Verification items for the finished model (mm, model axes). A direction names the side the tool comes from. Round coordinates to 2 decimals unless told otherwise and drop trailing zeros. Loops run counter-clockwise (first coordinate to the right, second up) from the corner with the lowest first, then second, coordinate; pieces in that order, holes last. Notation, with made-up numbers: M -27,-28.75 L -12,-28.75 A19 ccw -12,-21.75 Z; hole C -40,28.25 d10. An arc over 180 degrees is marked long. Write item = value, one per line. Start each with the question number.
Autodesk Inventor part; units mm, degrees
ref_plane "YZ Plane" through (0, 0, 0) normal (1, 0, 0) x (0, 1, 0)
ref_plane "XZ Plane" through (0, 0, 0) normal (0, 1, 0) x (-1, 0, 0)
ref_plane "XY Plane" through (0, 0, 0) normal (0, 0, 1) x (1, 0, 0)
sketch "Skizze1" plane through (0, 0, 0) normal (0, 0, 1) x (1, 0, 0)
  arc A0 (-19, -51.1238) -> (19, -51.1238) centre (0, -51.1238) ccw
  line L0 (-19, -72.2231) -> (-19, -51.1238)
  line L1 (-19, -72.2231) -> (-29, -72.2231)
  line L2 (-29, -72.2231) -> (-29, -77.2231)
  line L3 (29, -77.2231) -> (-29, -77.2231)
  line L4 (29, -77.2231) -> (29, -72.2231)
  line L5 (29, -72.2231) -> (19, -72.2231)
  line L6 (19, -72.2231) -> (19, -51.1238)
  circle A1 centre (0, -47.6238) radius 17.5
  circle A2 centre (0, -40.6238) radius 6
  arc A3 (19, -46.6238) -> (-19, -46.6238) centre (0, -46.6238) ccw
  line L7 (-19, -46.6238) -> (-19, -51.1238)
  line L8 (19, -46.6238) -> (19, -51.1238)
  circle A4 centre (-13.446, -71.669) radius 2.1
  circle A5 centre (13.446, -71.669) radius 2.1
  point P0 (0, 0)
extrude "Extrusion1" add sketch "Skizze1" along normal blind 8 contours L7 A3 L8 A0 | A0 L6 L5 L4 L3 L2 L1 L0 | A1 | A4 | A5
sketch "Skizze2" plane through (-29, -77.2231, 0) normal (0, -1, 0) x (1, 0, 0)
  circle A0 centre (4, 4.5) radius 2.35
  circle A1 centre (54, 4.5) radius 2.35
  point P0 (29, 0)
hole "Bohrung1" at (-25, -77.2231, 4.5) at (25, -77.2231, 4.5) direction (0, 1, 0) diameter 4 end through all
sketch "Skizze3" plane through (0, 0, 0) normal (0, 0, -1) x (-1, 0, 0)
  circle A0 centre (0, -40.6238) radius 6
  line L0 (-19, -72.2231) -> (-19, -46.6238)
  line L1 (-29, -72.2231) -> (-19, -72.2231)
  line L2 (-29, -77.2231) -> (-29, -72.2231)
  line L3 (29, -77.2231) -> (-29, -77.2231)
  line L4 (29, -72.2231) -> (29, -77.2231)
  line L5 (19, -72.2231) -> (29, -72.2231)
  line L6 (19, -46.6238) -> (19, -72.2231)
  arc A1 (19, -46.6238) -> (-19, -46.6238) centre (0, -46.6238) ccw
  point P0 (0, 0)
extrude "Extrusion2" cut sketch "Skizze3" against normal blind 0.5
sketch "Skizze4" plane through (0, 0, 8) normal (0, 0, 1) x (1, 0, 0)
  circle A0 centre (-13.446, -71.669) radius 2.1
  circle A1 centre (13.446, -71.669) radius 2.1
  point P0 (0, 0)
hole "Bohrung2" at (-13.446, -71.669, 8) at (13.446, -71.669, 8) direction (0, 0, -1) diameter 4 end through all
sketch "Skizze5" plane through (0, 0, 0.5) normal (0, 0, -1) x (-1, 0, 0)
  circle A0 centre (13.446, -71.669) radius 2
  circle A1 centre (-13.446, -71.669) radius 2
  line L0 (-19, -72.2231) -> (-19, -46.6238)
  line L1 (19, -46.6238) -> (19, -72.2231)
  line L2 (-13.446, -67.6276) -> (-9.946, -69.6483)
  line L3 (-9.946, -69.6483) -> (-9.946, -73.6898)
  line L4 (-9.946, -73.6898) -> (-13.446, -75.7105)
  line L5 (-13.446, -75.7105) -> (-16.946, -73.6898)
  line L6 (-16.946, -73.6898) -> (-16.946, -69.6483)
  line L7 (-16.946, -69.6483) -> (-13.446, -67.6276)
  line L8 (13.446, -67.6276) -> (16.946, -69.6483)
  line L9 (16.946, -69.6483) -> (16.946, -73.6898)
  line L10 (16.946, -73.6898) -> (13.446, -75.7105)
  line L11 (13.446, -75.7105) -> (9.946, -73.6898)
  line L12 (9.946, -73.6898) -> (9.946, -69.6483)
  line L13 (9.946, -69.6483) -> (13.446, -67.6276)
  point P0 (0, 0)
  dimension "d18" = 7
extrude "Extrusion3" cut sketch "Skizze5" against normal blind 3 contours A0 | A1 | L2 L3 L4 L5 L6 L7 | L8 L9 L10 L11 L12 L13
sketch "Skizze8" plane through (0, 0, 8) normal (0, 0, 1) x (1, 0, 0)
  circle A0 centre (0, -40.6238) radius 6
  line L0 (-29, -77.2231) -> (29, -77.2231)
  circle A1 centre (0, -47.6238) radius 15.5 construction
  line L1 (0, -40.6238) -> (0, -77.2231) construction
  line L2 (-13.4234, -39.8738) -> (0, -47.6238) construction
  line L3 (0, -47.6238) -> (13.4234, -39.8738) construction
  line L4 (0, -47.6238) -> (0, -32.1238) construction
  point P0 (0, 0)
  point P1 (0, -63.1238)
  dimension "d21" = 31
  dimension "d22" = 7
  dimension "d23" = 60
hole "Bohrung3" at (-13.4234, -39.8738, 8) at (13.4234, -39.8738, 8) at (0, -63.1238, 8) direction (0, 0, -1) diameter 3.2 end through all counterbore diameter 6 counterbore depth 3
sketch "Skizze9" plane through (0, 0, 8) normal (0, 0, 1) x (1, 0, 0)
  circle A0 centre (0, -40.6238) radius 6
  circle A1 centre (0, -40.6238) radius 6.1
  point P0 (0, 0)
  dimension "d31" = 12.2
extrude "Extrusion4" cut sketch "Skizze9" against normal through all contours A0 | A1
sketch "Skizze10" plane through (0, 0, 3.5) normal (0, 0, -1) x (-1, 0, 0)
  circle A0 centre (13.446, -71.669) radius 2
  circle A1 centre (-13.446, -71.669) radius 2
  circle A2 centre (-13.446, -71.669) radius 2
  line L0 (-13.446, -67.6276) -> (-9.946, -69.6483)
  line L1 (-16.946, -69.6483) -> (-13.446, -67.6276)
  line L2 (-16.946, -73.6898) -> (-16.946, -69.6483)
  line L3 (-13.446, -75.7105) -> (-16.946, -73.6898)
  line L4 (-9.946, -73.6898) -> (-13.446, -75.7105)
  line L5 (-9.946, -69.6483) -> (-9.946, -73.6898)
  point P0 (0, 0)
extrude "Extrusion5" add sketch "Skizze10" against normal blind 0.2 contours A0 | A1
sketch "Skizze11" plane through (0, 0, 8) normal (0, 0, 1) x (1, 0, 0)
  circle A0 centre (0, -63.1238) radius 3
  arc A1 (19, -46.6238) -> (-19, -46.6238) centre (0, -46.6238) ccw
  arc A2 (15, -16.1238) -> (15, -21.1238) centre (15, -18.6238) ccw construction
  line L0 (15, -16.1238) -> (23, -16.1238) construction
  arc A3 (23, -21.1238) -> (23, -16.1238) centre (23, -18.6238) ccw construction
  line L1 (23, -21.1238) -> (15, -21.1238) construction
  arc A4 (-23, -16.1238) -> (-23, -21.1238) centre (-23, -18.6238) ccw construction
  line L2 (-23, -16.1238) -> (-15, -16.1238) construction
  arc A5 (-15, -21.1238) -> (-15, -16.1238) centre (-15, -18.6238) ccw construction
  line L3 (-15, -21.1238) -> (-23, -21.1238) construction
  line L4 (23, -25.6238) -> (-23, -25.6238) construction
  arc A6 (23, -25.6238) -> (23, -11.6238) centre (23, -18.6238) ccw construction
  line L5 (-23, -11.6238) -> (23, -11.6238) construction
  arc A7 (-23, -11.6238) -> (-23, -25.6238) centre (-23, -18.6238) ccw construction
  line L6 (-8, -29.3901) -> (8, -29.3901)
  line L7 (8, -29.3901) -> (8, -13.6238)
  line L8 (6, -11.6238) -> (-6, -11.6238)
  line L9 (-8, -13.6238) -> (-8, -29.3901)
  line L10 (0, -63.1238) -> (0, -11.6238) construction
  circle A8 centre (-15, -18.6238) radius 7 construction
  arc A9 (-6, -11.6238) -> (-8, -13.6238) centre (-6, -13.6238) ccw
  arc A10 (8, -13.6238) -> (6, -11.6238) centre (6, -13.6238) ccw
  line L11 (-8, -20.2888) -> (-16.9654, -38.0696)
  line L12 (8, -20.2888) -> (16.9654, -38.0696)
  circle A11 centre (0, -18.6238) radius 2
  point P0 (0, 0)
  point P1 (8, -11.6238)
  dimension "d36" = 2
extrude "Extrusion6" add sketch "Skizze11" against normal up to surface (7.5 mm away) contours A1 L7 L12 | A1 L9 A9 L8 A10 L7 | A1 L11 L9 | A11
fillet "Rundung1" radius 3 2 edges at (-8, -20.2888, 4.25) (8, -20.2888, 4.25)
sketch "Skizze12" plane through (0, 0, 0.5) normal (0, 0, -1) x (-1, 0, 0)
  circle A0 centre (0, -63.1238) radius 1.6
  line L0 (6, -11.6238) -> (-6, -11.6238)
  line L1 (-8, -13.6238) -> (-8, -19.5752)
  arc A1 (-23, -16.1238) -> (-23, -21.1238) centre (-23, -18.6238) ccw
  arc A2 (23, -21.1238) -> (23, -16.1238) centre (23, -18.6238) ccw
  line L2 (-23, -18.6238) -> (23, -18.6238) construction
  line L3 (0, -11.6238) -> (0, -63.1238) construction
  point P0 (0, 0)
  point P1 (0, -18.6238)
hole "Bohrung4" at (0, -18.6238, 0.5) direction (0, 0, 1) diameter 4 end through all
sketch "Skizze13" plane through (0, 0, 0.5) normal (0, 0, -1) x (-1, 0, 0)
  circle A0 centre (0, -18.6238) radius 2
  line L0 (-8, -13.6238) -> (-8, -19.5752)
  line L1 (0, -14.5824) -> (3.5, -16.6031)
  line L2 (3.5, -16.6031) -> (3.5, -20.6446)
  line L3 (3.5, -20.6446) -> (0, -22.6653)
  line L4 (0, -22.6653) -> (-3.5, -20.6446)
  line L5 (-3.5, -20.6446) -> (-3.5, -16.6031)
  line L6 (-3.5, -16.6031) -> (0, -14.5824)
  point P0 (0, 0)
  dimension "d47" = 7
extrude "Extrusion7" cut sketch "Skizze13" against normal blind 3 contours A0 | L1 L2 L3 L4 L5 L6
sketch "Skizze14" plane through (0, 0, 3.5) normal (0, 0, -1) x (-1, 0, 0)
  circle A0 centre (0, -18.6238) radius 2
  point P0 (0, 0)
extrude "Extrusion8" add sketch "Skizze14" against normal blind 0.2
properties part number "EllbowMotorMount" material "ABS-Kunststoff - Schwarz"
1. Section check A-A, the plane x = -25. Enter the section's corners in (y, z).
2. Tool access check on faces 1 (the flat face through (11.671, -74.686, 1.979)), 2 (the flat face through (-8, -17, 4)), 3 (the flat face through (12.583, -29.378, 4.302)), 4 (the flat face through (-12, -41, 5)). Record the directions out of +Z, -Z, +X, -X, +Y, -Y that give a thin tool (end or side, any length) a straight path to the whole face; none if there is none.
3. Mould release check, pull along Y, two halves, no side actions. Record for faces 5 (the cylindrical face through (-18.5, -42.3, 4.2)), 6 (the cylindrical face through (13.36, -69.67, 5.82)), 7 (the cylindrical face through (26.2, -74.7, 6.1)): pulls with the +Y half, pulls with the -Y half, needs draft (parallel to the pull), parting line crosses it, or undercut.
4. Section check C-C, the plane z = 1.25. Give the number of separate pieces and of enclosed holes in the cut face, and give its area (3 significant figures).
5. Section check B-B, the plane y = -39. Enter the section's corners in (x, z).
6. Gauge pin test, flat ends, axial feed: P1, Ø2, axis at x = 14, y = -71.5, coming from the +Z side; P2, Ø1, axis at x = 16, z = 3.5, coming from the +Y side; P3, Ø1.8, axis at x = 15, y = -41, coming from the +Z side. Record the tip position at first contact, or that the pin passes through.
7. Thickness scan on line 1 (Y direction, x = 0, z = 2); line 2 (Z direction, x = -25, y = -74); line 3 (Y direction, x = -2.5, z = 7). Record the ranges inside material, lowest first.
8. Section check D-D, the plane y = -70.5. Enter the section's corners in (x, z).
Computed values:
q1.outline = M -77.22,0.5 L -72.22,0.5 L -72.22,2.5 L -77.22,2.5 Z; M -77.22,6.5 L -72.22,6.5 L -72.22,8 L -77.22,8 Z
q2.face_1 = -Z
q2.face_2 = +Z, -Z, -X, +Y
q2.face_3 = +Z, -Z, +X, +Y
q2.face_4 = +Z
q3.face_5 = pulls with the +Y half
q3.face_6 = undercut
q3.face_7 = needs draft
q4.separate_pieces = 1
q4.enclosed_holes = 7
q4.area = 1,890 mm2
q5.outline = M -17.4,0.5 L -14.76,0.5 L -14.76,5 L -16.29,5 L -16.29,8 L -17.4,8 Z; M -12.08,0.5 L -5.88,0.5 L -5.88,8 L -10.55,8 L -10.55,5 L -12.08,5 Z; M 5.88,0.5 L 12.08,0.5 L 12.08,5 L 10.55,5 L 10.55,8 L 5.88,8 Z; M 14.76,0.5 L 17.4,0.5 L 17.4,8 L 16.29,8 L 16.29,5 L 14.76,5 Z
q6.P1 = 3.7
q6.P2 = -35.16
q6.P3 = 5
q7.line_1 = -77.22 to -64.72, -61.52 to -46.72, -34.52 to -22.67, -14.58 to -11.62
q7.line_2 = 0.5 to 2.5, 6.5 to 8
q7.line_3 = -77.22 to -64.78, -61.47 to -46.19, -35.06 to -11.62
q8.outline = M -19,0.5 L -16.95,0.5 L -16.95,3.5 L -9.95,3.5 L -9.95,0.5 L 9.95,0.5 L 9.95,3.5 L 16.95,3.5 L 16.95,0.5 L 19,0.5 L 19,8 L 15.07,8 L 15.07,3.7 L 11.82,3.7 L 11.82,8 L -11.82,8 L -11.82,3.7 L -15.07,3.7 L -15.07,8 L -19,8 Z
